Read the model definition and answer for the solid it produces. Units are mm, in the model's axes. A direction names the side the tool comes from. Coordinates: 2 decimals unless noted, no trailing zeros. Loops run counter-clockwise (first coordinate to the right, second up) from the corner with the lowest first, then second, coordinate; pieces in that order, holes last.
from build123d import *

# Parameters (mm, degrees)
SKETCH2_W                                           = 70
SKETCH2_H                                           = 86
BOSS_EXTRUDE1_DEPTH                                 = 35
CUT_EXTRUDE1_DEPTH                                  = 26
SKETCH2_3_R                                         = 12.75
BOSS_EXTRUDE2_DEPTH                                 = 9
SKETCH3_3_R                                         = 11
SKETCH3_3_R_2                                       = 5
CUT_EXTRUDE2_DEPTH                                  = 28
SKETCH3_4_R                                         = 5
CUT_EXTRUDE3_DEPTH                                  = 171.076453397
SKETCH15_R                                          = 13.5
CUT_EXTRUDE4_DEPTH                                  = 4
CBORE_FOR_M3_HEX_SOCKET_HEAD_CAP_SCREW1_D           = 3.6
CBORE_FOR_M3_HEX_SOCKET_HEAD_CAP_SCREW1_CBORE_D     = 6.5
CBORE_FOR_M3_HEX_SOCKET_HEAD_CAP_SCREW1_CBORE_DEPTH = 3.4
F_4_6_4_6_DIAMETER_HOLE1_D                          = 4.6
F_4_6_4_6_DIAMETER_HOLE1_DEPTH                      = 6
F_4_6_4_6_DIAMETER_HOLE1_TIP                        = 1.381979424
CBORE_FOR_M3_HEX_SOCKET_HEAD_CAP_SCREW2_D           = 3.4
CBORE_FOR_M3_HEX_SOCKET_HEAD_CAP_SCREW2_CBORE_D     = 6.5
CBORE_FOR_M3_HEX_SOCKET_HEAD_CAP_SCREW2_CBORE_DEPTH = 3.4
F_4_6_4_6_DIAMETER_HOLE2_D                          = 4.6
F_4_6_4_6_DIAMETER_HOLE2_DEPTH                      = 6
F_4_6_4_6_DIAMETER_HOLE2_TIP                        = 1.381979424
F_4_6_4_6_DIAMETER_HOLE3_D                          = 4.6
F_4_6_4_6_DIAMETER_HOLE3_DEPTH                      = 5
F_4_6_4_6_DIAMETER_HOLE3_TIP                        = 1.381979424
SKETCH19_W                                          = 7
SKETCH19_H                                          = 43
CUT_EXTRUDE5_DEPTH                                  = 7
F_2_5MM_CHAMFER1_SIZE                               = 2.5
F_0_5MM_CHAMFER2_SIZE                               = 0.5


with BuildPart() as part:
    # Sketch2 → Boss-Extrude1 (new body)
    with BuildSketch(Plane(origin=(0, 0, 0), x_dir=(0, 0, -1), z_dir=(1, 0, 0))):
        with Locations((35, 43)):
            Rectangle(SKETCH2_W, SKETCH2_H)
    extrude(amount=BOSS_EXTRUDE1_DEPTH)

    # Sketch3 → Cut-Extrude1 (cut)
    with BuildSketch(Plane(origin=(35, 0, 0), x_dir=(0, 0, -1), z_dir=(1, 0, 0))):
        Polygon((13.5, 0), (56.5, 0), (56.5, 86), (13.5, 86), (13.5, 73), (3.5, 73), (3.5, 56), (13.5, 56), align=None)
    extrude(amount=-CUT_EXTRUDE1_DEPTH, mode=Mode.SUBTRACT)

    # Sketch2<3> → Boss-Extrude2 (add)
    with BuildSketch(Plane(origin=(0, 0, 0), x_dir=(0, 0, -1), z_dir=(1, 0, 0))):
        with BuildLine():
            Line((0, 116), (0, 86))
            Line((0, 86), (70, 86))
            Line((70, 86), (70, 116))
            ThreePointArc((70, 116), (35, 151), (0, 116))
        make_face()
        with Locations((35, 116)):
            Circle(SKETCH2_3_R, mode=Mode.SUBTRACT)
    extrude(amount=BOSS_EXTRUDE2_DEPTH)

    # Sketch3<3> → Cut-Extrude2 (cut)
    # profile 1 of 2: a face of its own
    with BuildSketch(Plane(origin=(35, 0, 0), x_dir=(0, 0, -1), z_dir=(1, 0, 0))):
        with Locations((35, 21.5)):
            Circle(SKETCH3_3_R)
        with Locations((35, 21.5)):
            Circle(SKETCH3_3_R_2, mode=Mode.SUBTRACT)
    # profile 2 of 2: a face of its own
    with BuildSketch(Plane(origin=(35, 0, 0), x_dir=(0, 0, -1), z_dir=(1, 0, 0))):
        with Locations((35, 21.5)):
            Circle(SKETCH3_3_R_2)
    extrude(amount=-CUT_EXTRUDE2_DEPTH, mode=Mode.SUBTRACT)

    # Sketch3<4> → Cut-Extrude3 (cut, through all)
    with BuildSketch(Plane(origin=(35, 0, 0), x_dir=(0, 0, -1), z_dir=(1, 0, 0))):
        with Locations((35, 21.5)):
            Circle(SKETCH3_4_R)
    extrude(amount=-CUT_EXTRUDE3_DEPTH, mode=Mode.SUBTRACT)

    # Sketch15 → Cut-Extrude4 (cut)
    with BuildSketch(Plane(origin=(9, 0, 0), x_dir=(0, 0, -1), z_dir=(1, 0, 0))):
        with Locations((35, 116)):
            Circle(SKETCH15_R)
    cut_extrude4 = extrude(amount=-CUT_EXTRUDE4_DEPTH, mode=Mode.SUBTRACT)

    # Mirror1: Cut-Extrude4 across plane
    add(cut_extrude4.mirror(Plane(origin=(4.5, 0, 0), x_dir=(0, 0, 1), z_dir=(1, 0, 0))), mode=Mode.SUBTRACT)

    # CBORE for M3 Hex Socket Head Cap Screw1 (through all)
    with Locations(Plane.ZY):
        with Locations((-19.5, 6), (-35, 21.5), (-19.5, 37), (-50.5, 6), (-50.5, 37)):
            CounterBoreHole(CBORE_FOR_M3_HEX_SOCKET_HEAD_CAP_SCREW1_D / 2, CBORE_FOR_M3_HEX_SOCKET_HEAD_CAP_SCREW1_CBORE_D / 2, CBORE_FOR_M3_HEX_SOCKET_HEAD_CAP_SCREW1_CBORE_DEPTH)

    # Ø4.6 (4.6) Diameter Hole1
    with Locations(Plane(origin=(0, 0, 0), x_dir=(-1, 0, 0), z_dir=(0, -1, 0))):
        with Locations((-4.5, 35), (-35, 35), (-4.5, 63.5), (-4.5, 6.5)):
            Hole(F_4_6_4_6_DIAMETER_HOLE1_D / 2, depth=F_4_6_4_6_DIAMETER_HOLE1_DEPTH)
            with Locations((0, 0, -(F_4_6_4_6_DIAMETER_HOLE1_DEPTH + F_4_6_4_6_DIAMETER_HOLE1_TIP / 2))):  # 118° drill point
                Cone(0, F_4_6_4_6_DIAMETER_HOLE1_D / 2, F_4_6_4_6_DIAMETER_HOLE1_TIP, mode=Mode.SUBTRACT)

    # CBORE for M3 Hex Socket Head Cap Screw2 (through all)
    with Locations(Plane.ZY):
        with Locations((-63.25, 81)):
            CounterBoreHole(CBORE_FOR_M3_HEX_SOCKET_HEAD_CAP_SCREW2_D / 2, CBORE_FOR_M3_HEX_SOCKET_HEAD_CAP_SCREW2_CBORE_D / 2, CBORE_FOR_M3_HEX_SOCKET_HEAD_CAP_SCREW2_CBORE_DEPTH)

    # Ø4.6 (4.6) Diameter Hole2
    with Locations(Plane(origin=(35, 0, 0), x_dir=(0, 0, -1), z_dir=(1, 0, 0))):
        with Locations((6.75, 81)):
            Hole(F_4_6_4_6_DIAMETER_HOLE2_D / 2, depth=F_4_6_4_6_DIAMETER_HOLE2_DEPTH)
            with Locations((0, 0, -(F_4_6_4_6_DIAMETER_HOLE2_DEPTH + F_4_6_4_6_DIAMETER_HOLE2_TIP / 2))):  # 118° drill point
                Cone(0, F_4_6_4_6_DIAMETER_HOLE2_D / 2, F_4_6_4_6_DIAMETER_HOLE2_TIP, mode=Mode.SUBTRACT)

    # Ø4.6 (4.6) Diameter Hole3
    with Locations(Plane.ZY):
        with Locations((-60, 68.75), (-10, 68.75)):
            Hole(F_4_6_4_6_DIAMETER_HOLE3_D / 2, depth=F_4_6_4_6_DIAMETER_HOLE3_DEPTH)
            with Locations((0, 0, -(F_4_6_4_6_DIAMETER_HOLE3_DEPTH + F_4_6_4_6_DIAMETER_HOLE3_TIP / 2))):  # 118° drill point
                Cone(0, F_4_6_4_6_DIAMETER_HOLE3_D / 2, F_4_6_4_6_DIAMETER_HOLE3_TIP, mode=Mode.SUBTRACT)

    # Sketch19 → Cut-Extrude5 (cut)
    with BuildSketch(Plane(origin=(0, 0, -13.5), x_dir=(-1, 0, 0), z_dir=(0, 0, -1))):
        with Locations((-31.5, 34.5)):
            Rectangle(SKETCH19_W, SKETCH19_H)
    extrude(amount=-CUT_EXTRUDE5_DEPTH, mode=Mode.SUBTRACT)

    # 2,5mm Chamfer1
    f_2_5mm_chamfer1_edges = [part.edges().sort_by_distance(p)[0] for p in [
        (0, 151, -35),
        (0, 58, 0),
        (0, 58, -70),
        (22, 86, 0),
        (22, 86, -70),
    ]]
    chamfer(f_2_5mm_chamfer1_edges, length=F_2_5MM_CHAMFER1_SIZE)

    # 0,5mm Chamfer2
    f_0_5mm_chamfer2_edges = [part.edges().sort_by_distance(p)[0] for p in [
        (9, 6, -48.7),
        (0, 6, -53.75),
        (9, 37, -17.7),
        (0, 37, -22.75),
        (2.2, 0, -35),
        (2.2, 0, -6.5),
        (2.2, 0, -63.5),
        (0, 81, -66.5),
        (35, 81, -61.55),
        (35, 81, -9.05),
        (0, 68.75, -57.7),
        (0, 68.75, -7.7),
        (22, 86, -13.5),
        (22, 86, -56.5),
        (9, 99.75, 0),
        (9, 99.75, -70),
        (9, 151, -35),
        (9, 21.5, -24),
        (7, 21.5, -30),
        (0, 21.5, -30),
        (9, 116, -21.5),
        (0, 116, -21.5),
        (9, 6, -17.7),
        (0, 6, -22.75),
        (9, 37, -48.7),
        (0, 37, -53.75),
    ]]
    chamfer(f_0_5mm_chamfer2_edges, length=F_0_5MM_CHAMFER2_SIZE)


solid = part.part
Item 1: A cutting plane is placed at C-C on y = 37. Give the number of separate pieces and of enclosed holes in the cut face, then the cut area to 3 significant figures.
Numbers:
separate pieces: 3
enclosed holes: 0
area: 1,190 mm2
Item 2: Determine the mould class of faces 4 (the face through (4.49, 128.64, -33.34)), 5 (the face through (3.4, 35.6, -49.1)), 6 (the face through (4.55, 7.14, -6.9)) for opening direction X: released by +X, released by -X, zero draft, split by the parting line, or undercut.
Numbers:
face 4: zero draft
face 5: released by -X
face 6: undercut
Item 3: A cutting plane is placed at B-B on y = 96. Determine the outline of the cut face in (x, z), then the cut area to 4 significant figures.
Numbers:
outline: (0, -67.5) - (2.5, -70) - (8.5, -70) - (9, -69.5) - (9, -0.5) - (8.5, 0) - (2.5, 0) - (0, -2.5) - close
area: 623.5 mm2
Item 4: Which of the six approach directions +Z, -Z, +X, -X, +Y, -Y give full straight-line access (tool end or side, diameter ignored) to faces 1 (the face through (31.712, 78.755, -7.249)), 2 (the face through (2.226, 120.055, -47.877)), 3 (the face through (22, 42, -56.5))?
Numbers:
face 1: +X
face 2: -X
face 3: +X, +Y, -Y
Item 5: A cutting plane is placed at A-A on x = 22.5. Determine the outline of the cut face in (y, z).
Numbers:
outline: (0, -70) - (83.5, -70) - (86, -67.5) - (86, -57) - (85.5, -56.5) - (0, -56.5) - close; (0, -13.5) - (56, -13.5) - (56, -3.5) - (73, -3.5) - (73, -13.5) - (85.5, -13.5) - (86, -13) - (86, -2.5) - (83.5, 0) - (0, 0) - close; hole circle Ø3.4 at (81, -63.25)
Item 6: Find the intervals of material crossed by line 1 along Y through (x, z) = (30, -6); line 2 along Z through (x, y) = (21.5, 27.5); line 3 along Z through (x, y) = (1, 70.5), in increasing order.
Numbers:
line 1: y = 0 to 56, 73 to 78.83, 83.17 to 86
line 2: z = -70 to -56.5, -13.5 to 0
line 3: z = -68.5 to -61.49, -58.51 to -11.49, -8.51 to -1.5
Item 7: Given pin 1 (6 mm diameter, centred on x = 4.5, z = -35, fed in from -Y); pin 2 (3 mm diameter, centred on y = 36, z = -50.5, fed in from -X); pin 3 (5.5 mm diameter, centred on x = 22.5, z = -8, fed in from +Y); pin 4 (16 mm diameter, centred on y = 21.5, z = -35, fed in from +X), each flat-ended and moving along its own axis, determine where each tip first touches the part or whether it passes through.
Numbers:
pin 1: stops at y = 0
pin 2: stops at x = 3.4
pin 3: stops at y = 86
pin 4: stops at x = 7
